Check sheet for the drawn part. Datum: minimum x, y, z corner. Units: mm. A direction names the side the tool comes from. Give positions to 0.01 mm unless a question says otherwise; leave off trailing zeros. Order: outer loops, then holes, each group sorted by start corner. A loop starts at its lowest first (then second) coordinate and runs counter-clockwise, first axis right, second up. Notation, with made-up numbers: (17.25, 45.5) -> (76.25, 45.5) arc R24 ccw to (76.25, 73.5) -> close; hole circle Ø10 at (30, 74). An arc over 180 degrees is marked (long way). One line per question, with ' | ' between items. Start each with the question number.
Q1. Access from +Z, -Z, +X, -X, +Y, -Y to the whole of each face (thin tool, end or side, straight path). Record for the marked faces 1, 2 and 3.
Q2. Section check A-A on y = 6.8. Record the cut outline in (x, z), plus the area to 3 significant figures.
Q3. Mould release check, pull along X, two halves, no side actions. Record for the marked faces 4, 5 and 6: released by +X, released by -X, zero draft, split by the parting line, or undercut.
Q4. Section check C-C on z = 1.3. Record the cut outline in (x, y).
Q5. Material ranges on probe 1 along Y at (x, z) = (6.8, 3.6); probe 2 along Y at (x, z) = (6.8, 1.3); probe 3 along Z at (x, y) = (10, 5), recorded low to high. Write a range as [from, to].
Q6. Go/stop test with flat-tipped pins: pin 1 (2 mm diameter, centred on y = 10, z = 2.5, fed in from +X); pin 2 (5.5 mm diameter, centred on x = 6.8, y = 6.8, fed in from +Z). Record where each tip stops, or that it passes through.
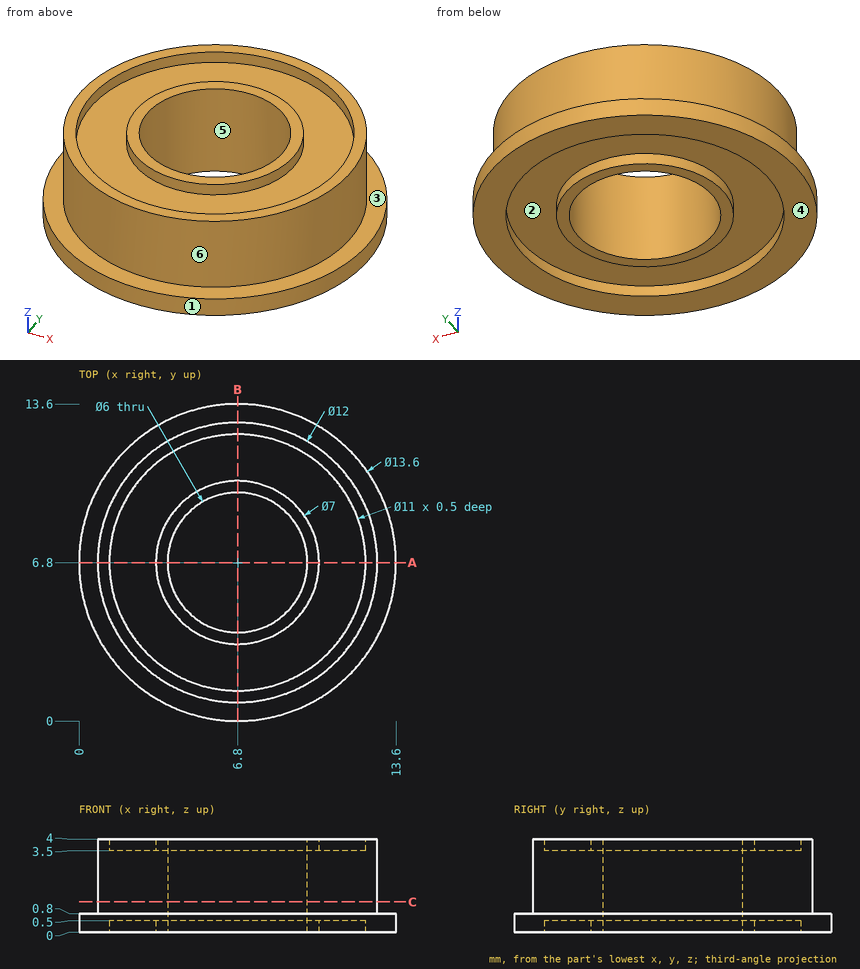
Filled in:
1) face 1: +Z, -Z | face 2: -Z | face 3: +Z
2) outline: (0, 0) -> (1.3, 0) -> (1.3, 0.5) -> (3.3, 0.5) -> (3.3, 0) -> (3.8, 0) -> (3.8, 4) -> (3.3, 4) -> (3.3, 3.5) -> (1.3, 3.5) -> (1.3, 4) -> (0.8, 4) -> (0.8, 0.8) -> (0, 0.8) -> close; (9.8, 0) -> (10.3, 0) -> (10.3, 0.5) -> (12.3, 0.5) -> (12.3, 0) -> (13.6, 0) -> (13.6, 0.8) -> (12.8, 0.8) -> (12.8, 4) -> (12.3, 4) -> (12.3, 3.5) -> (10.3, 3.5) -> (10.3, 4) -> (9.8, 4) -> close | area: 21.3 mm²
3) face 4: zero draft | face 5: undercut | face 6: split by the parting line
4) outline: circle Ø12 at (6.8, 6.8); hole circle Ø6 at (6.8, 6.8)
5) probe 1: [0.8, 1.3], [3.3, 3.8], [9.8, 10.3], [12.3, 12.8] | probe 2: [0.8, 3.8], [9.8, 12.8] | probe 3: [0.5, 3.5]
6) pin 1: x = 12.38 | pin 2: through
